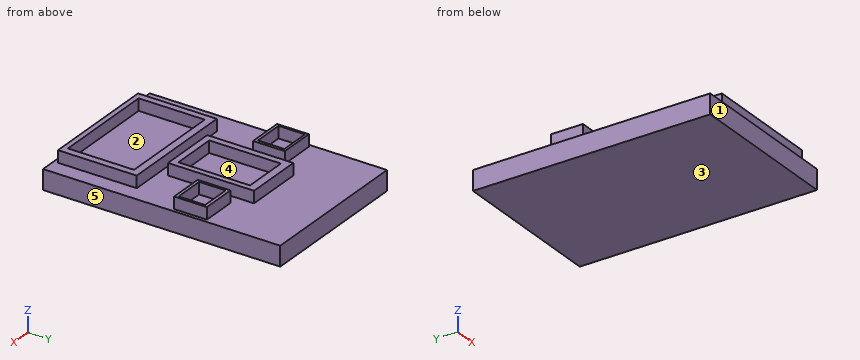
from build123d import *

# Parameters (mm, degrees)
F0_W     = 101.6
F0_H     = 152.4
F0_W_2   = 25.9637702256
F0_H_2   = 38.2640473545
F1_DEPTH = 12.7
F2_W     = 37.3481158167
F2_H     = 55.3146842867
F2_W_2   = 29.3511133641
F2_H_2   = 46.0022222251
F2_W_3   = 76.2175656855
F2_H_3   = 50.5883861333
F2_W_4   = 67.3006474972
F2_H_4   = 42.5056517124
F2_W_5   = 22.4156714976
F2_H_5   = 21.067361813
F2_W_6   = 19.5578802377
F2_H_6   = 17.0068526641
F2_W_7   = 22.81752415
F2_H_7   = 20.4082219861
F3_DEPTH = 7.62


with BuildPart() as f1:
    # F0 (on Top) → F1 (new body)
    with BuildSketch(Plane.XY):
        with Locations((-0.5644435562, 0)):
            Rectangle(F0_W, F0_H)
        with Locations((0.3079539165, 19.1320236772)):
            Rectangle(F0_W_2, F0_H_2, mode=Mode.SUBTRACT)
        with Locations((0.3079539165, 19.1320236772)):
            Rectangle(F0_W_2, F0_H_2)
    extrude(amount=F1_DEPTH)

    # F2 (on face) → F3 (join)
    with BuildSketch(Plane.XY.offset(12.7)):
        with Locations((0.2927491441, 10.6312921271)):
            Rectangle(F2_W, F2_H)
        with Locations((0.5644438788, 10.1600000635)):
            Rectangle(F2_W_2, F2_H_2, mode=Mode.SUBTRACT)
        with Locations((1.8496308476, -48.2227718458)):
            Rectangle(F2_W_3, F2_H_3)
        with Locations((1.7533935606, -48.9725470543)):
            Rectangle(F2_W_4, F2_H_4, mode=Mode.SUBTRACT)
        with Locations((36.8676688522, 17.0947427396)):
            Rectangle(F2_W_5, F2_H_5)
        with Locations((36.8869742379, 16.9948018156)):
            Rectangle(F2_W_6, F2_H_6, mode=Mode.SUBTRACT)
        with Locations((-38.0652910098, 17.0451246668)):
            Rectangle(F2_W_7, F2_H_7)
        with Locations((-38.3849483915, 17.1790141612)):
            Rectangle(F2_W_6, F2_H_6, mode=Mode.SUBTRACT)
    extrude(amount=F3_DEPTH)


solid = f1.part
Check sheet for the modelled part. Datum: model origin and axes. Units: mm. Face numbers are marked on the shaded views. A direction names the side the tool comes from. Give positions to 0.01 mm unless a question says otherwise; leave off trailing zeros. Loops run counter-clockwise (first coordinate to the right, second up) from the corner with the lowest first, then second, coordinate; pieces in that order, holes last. Notation, with made-up numbers: M -30.75,88 L -14.75,88 A19 ccw -14.75,93 Z; hole C 25,66 d4. An arc over 180 degrees is marked long. Answer as a JSON object with one key per item and string values. Group by question number.
Q1. Material ranges on line 1 along Y through (x, z) = (34, 14); line 2 along X through (y, z) = (21, 17); line 3 along Y through (x, z) = (40, 14), recorded low to high. Write a range as [from, to].
Q2. Access from +Z, -Z, +X, -X, +Y, -Y to the whole of each face (thin tool, end or side, straight path). Record for the marked faces 4 and 5.
Q3. Cross-section at D-D on x = -10. Record the cut outline in (y, z), then the cut area to 3 significant figures.
Q4. Cross-section at B-B on x = -34. Record the cut outline in (y, z), then the cut area to 3 significant figures.
Q5. Go/stop test with flat-tipped pins: P1, Ø6, axis at x = 5, z = 17, coming from the -Y side; P2, Ø8.5, axis at y = 17.5, z = 17, coming from the +X side; P3, Ø6, axis at x = 17.5, z = 17, coming from the +Y side; P4, Ø6, axis at y = 12, z = 15.5, coming from the -X side. Record where each tip stops, or that it passes through.
Q6. Release check for a two-part mould opening along Y. For the marked faces 1, 2 and 3 record: released by +Y, released by -Y, zero draft, split by the parting line, or undercut.
Q7. Cross-section at C-C on y = 29.5. Record the cut outline in (x, z), then the cut area to 3 significant figures.
Q8. Cross-section at A-A on z = 14.5. Give the number of separate pieces and of enclosed holes in the cut face, then the cut area to 3 significant figures.
Evaluation:
{
 "1": {"line 1": "y = [-73.52, -70.23], [-27.72, -22.93], [6.56, 8.49], [25.5, 27.63]", "line 2": "x = [-49.47, -48.16], [-28.61, -26.66], [-18.38, -14.11], [15.24, 18.97], [25.66, 27.11], [46.67, 48.08]", "line 3": "y = [6.56, 8.49], [25.5, 27.63]"},
 "2": {"face 4": "+Z", "face 5": "+Z, -Z, +X, +Y, -Y"},
 "3": {"outline": "M -76.2,0 L 76.2,0 L 76.2,12.7 L 38.29,12.7 L 38.29,20.32 L 33.16,20.32 L 33.16,12.7 L -12.84,12.7 L -12.84,20.32 L -17.03,20.32 L -17.03,12.7 L -22.93,12.7 L -22.93,20.32 L -27.72,20.32 L -27.72,12.7 L -70.23,12.7 L -70.23,20.32 L -73.52,20.32 L -73.52,12.7 L -76.2,12.7 Z", "area": "2,070 mm2"},
 "4": {"outline": "M -76.2,0 L 76.2,0 L 76.2,12.7 L 27.25,12.7 L 27.25,20.32 L 25.68,20.32 L 25.68,12.7 L 8.68,12.7 L 8.68,20.32 L 6.84,20.32 L 6.84,12.7 L -22.93,12.7 L -22.93,20.32 L -73.52,20.32 L -73.52,12.7 L -76.2,12.7 Z", "area": "2,350 mm2"},
 "5": {"P1": "stops at y = -73.52", "P2": "stops at x = 48.08", "P3": "stops at y = 38.29", "P4": "stops at x = -51.36"},
 "6": {"face 1": "released by -Y", "face 2": "undercut", "face 3": "zero draft"},
 "7": {"outline": "M -51.36,0 L 50.24,0 L 50.24,12.7 L 18.97,12.7 L 18.97,20.32 L 15.24,20.32 L 15.24,12.7 L -14.11,12.7 L -14.11,20.32 L -18.38,20.32 L -18.38,12.7 L -51.36,12.7 Z", "area": "1,350 mm2"},
 "8": {"separate pieces": "4", "enclosed holes": "4", "area": "1,980 mm2"}
}
